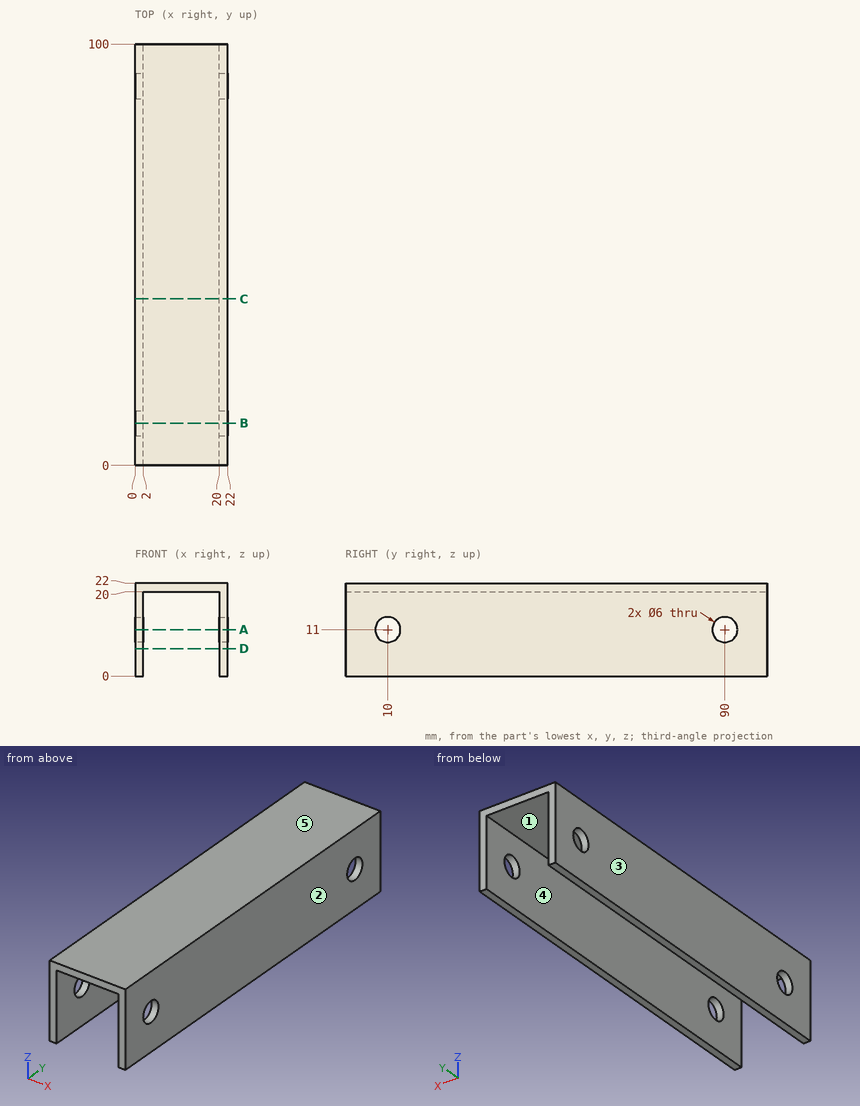
Job drawing, mm, ordinate dimensions from the low corner. One solid piece. A direction names the side the tool comes from. Give positions to 0.01 mm unless a question says otherwise; leave off trailing zeros. Order: outer loops, then holes, each group sorted by start corner. A loop starts at its lowest first (then second) coordinate and runs counter-clockwise, first axis right, second up. Notation, with made-up numbers: (12.25, 80) - (70.25, 80) arc R25 ccw to (70.25, 111) - close; hole circle Ø3 at (-9, -37). An arc over 180 degrees is marked (long way). Answer in a Markdown table with one row per item.
1. Tool access for the marked faces 4 and 5: list every direction of +Z, -Z, +X, -X, +Y, -Y with a clear straight run to the whole face (end or side of a thin tool).
Data:
| item | result |
|---|---|
| face 4 | -Z, +Y, -Y |
| face 5 | +Z, +X, -X, +Y, -Y |
2. Saw through at C-C, the plane y = 39.5. Give the cut face in (x, z), plus the area to 3 significant figures.
Data:
| item | result |
|---|---|
| outline | (0, 0) - (2, 0) - (2, 20) - (20, 20) - (20, 0) - (22, 0) - (22, 22) - (0, 22) - close |
| area | 124 mm² |
3. Saw through at A-A, the plane z = 11. Give the cut face in (x, y).
Data:
| item | result |
|---|---|
| outline | (0, 0) - (2, 0) - (2, 7) - (0, 7) - close; (0, 13) - (2, 13) - (2, 87) - (0, 87) - close; (0, 93) - (2, 93) - (2, 100) - (0, 100) - close; (20, 0) - (22, 0) - (22, 7) - (20, 7) - close; (20, 13) - (22, 13) - (22, 87) - (20, 87) - close; (20, 93) - (22, 93) - (22, 100) - (20, 100) - close |
4. Saw through at D-D, the plane z = 6.5. Give the cut face in (x, y), plus the area to 3 significant figures.
Data:
| item | result |
|---|---|
| outline | (0, 0) - (2, 0) - (2, 100) - (0, 100) - close; (20, 0) - (22, 0) - (22, 100) - (20, 100) - close |
| area | 400 mm² |
5. Saw through at B-B, the plane y = 10. Give the cut face in (x, z), plus the area to 3 significant figures.
Data:
| item | result |
|---|---|
| outline | (0, 0) - (2, 0) - (2, 8) - (0, 8) - close; (0, 14) - (2, 14) - (2, 20) - (20, 20) - (20, 14) - (22, 14) - (22, 22) - (0, 22) - close; (20, 0) - (22, 0) - (22, 8) - (20, 8) - close |
| area | 100 mm² |
6. Pull direction X, two halves, no side cores. Call the marked faces 1, 2 and 3: pulls with the +X half, pulls with the -X half, needs draft (parallel to the pull), parting line crosses it, or undercut.
Data:
| item | result |
|---|---|
| face 1 | undercut |
| face 2 | pulls with the +X half |
| face 3 | pulls with the -X half |
7. Flat gauge pins, fed straight in: pin 1 (12 mm diameter, centred on x = 9, z = 13, fed in from -Y); pin 2 (8 mm diameter, centred on y = 90, z = 11, fed in from -X). Where does each tip first touch, or does it go through?
Data:
| item | result |
|---|---|
| pin 1 | passes through |
| pin 2 | stops at x = 0 |
8. Probe probe 1 along Y at (x, z) = (0.85, 11); probe 2 along X at (y, z) = (25, 3.25); probe 3 along Z at (x, y) = (3, 15). List the from-to ranges inside material, lowest first. Write a range as [from, to].
Data:
| item | result |
|---|---|
| probe 1 | y = [0, 7], [13, 87], [93, 100] |
| probe 2 | x = [0, 2], [20, 22] |
| probe 3 | z = [20, 22] |
